```python
from build123d import *

# Parameters (mm, degrees)
ESBO_O1_W                     = 38
ESBO_O1_H                     = 56
ESBO_O1_R                     = 4
RESSALTO_EXTRUS_O1_DEPTH      = 6.4
ESBO_O6_R                     = 16.54
CORTE_EXTRUS_O5_DEPTH         = 4.6
ESBO_O7_R                     = 4
ESBO_O7_R_2                   = 1.25
CORTE_EXTRUS_O6_DEPTH         = 60.314079273
RESSALTO_EXTRUS_O2_DEPTH      = 4.6
RESSALTO_EXTRUS_O3_DEPTH      = 5.59
ESBO_O17_R                    = 3.5
RESSALTO_EXTRUS_O4_DEPTH      = 7
ESBO_O18_R                    = 2
RESSALTO_EXTRUS_O5_DEPTH      = 4
CHANFRO1_SIZE                 = 4
CHANFRO1_SIZE_2               = 5.29
FURO_ROSCADO_DE_M3X0_51_D     = 2.5
FURO_ROSCADO_DE_M3X0_51_DEPTH = 10
FURO_ROSCADO_DE_M3X0_51_TIP   = 0.751075774
CHANFRO2_SIZE                 = 1
SKETCH1_R                     = 1.25
CUT_EXTRUDE1_DEPTH            = 6
SKETCH2_R                     = 1.25
CUT_EXTRUDE2_DEPTH            = 10


# Read off the part's stored shape, not the designer's step: Escareado para parafuso de máquina com cabeça chata de M2.51
with BuildPart() as part:
    # Esboço1 → Ressalto-extrusão1 (new body)
    with BuildSketch(Plane.XY):
        with Locations((0, 28)):
            Rectangle(ESBO_O1_W, ESBO_O1_H)
        with Locations((0, 20)):
            Circle(ESBO_O1_R, mode=Mode.SUBTRACT)
    extrude(amount=RESSALTO_EXTRUS_O1_DEPTH)

    # Esboço6 → Corte-extrusão5 (cut)
    with BuildSketch(Plane(origin=(0, 0, 0), x_dir=(-1, 0, 0), z_dir=(0, 0, -1))):
        with Locations((0, 38.5)):
            Circle(ESBO_O6_R)
    extrude(amount=-CORTE_EXTRUS_O5_DEPTH, mode=Mode.SUBTRACT)

    # Esboço7 → Corte-extrusão6 (cut, through all)
    with BuildSketch(Plane(origin=(0, 0, 4.6), x_dir=(-1, 0, 0), z_dir=(0, 0, -1))):
        with Locations((0, 38.5)):
            Circle(ESBO_O7_R)
        with Locations((11.258330249, 32)):
            Circle(ESBO_O7_R_2)
        with Locations((-11.258330249, 32)):
            Circle(ESBO_O7_R_2)
        with Locations((0, 51.5)):
            Circle(ESBO_O7_R_2)
    extrude(amount=-CORTE_EXTRUS_O6_DEPTH, mode=Mode.SUBTRACT)

    # Escareado para parafuso de m_quina c 2 → Escareado para parafuso de máquina com cabeça chata de M2.51 (revolve, cut)
    with BuildSketch(Plane(origin=(-11.258330249, 32, 0), x_dir=(1, 0, 0), z_dir=(0, -1, 0))):
        Polygon((1.25, 4.6), (1.45, 4.6), (1.45, 5.1), (2.75, 6.4), (1.25, 6.4), align=None)
    revolve(axis=Axis((-11.258330249, 32, 0), (0, 0, 1)), mode=Mode.SUBTRACT)

    # Escareado para parafuso de m_quina c 3 o → Escareado para parafuso de m_quina c 3 (revolve, cut)
    with BuildSketch(Plane(origin=(11.258330249, 32, 0), x_dir=(1, 0, 0), z_dir=(0, -1, 0))):
        Polygon((1.25, 4.6), (1.45, 4.6), (1.45, 5.1), (2.75, 6.4), (1.25, 6.4), align=None)
    revolve(axis=Axis((11.258330249, 32, 0), (0, 0, 1)), mode=Mode.SUBTRACT)

    # Escareado para parafuso de m_quina c 4 o → Escareado para parafuso de m_quina c 4 (revolve, cut)
    with BuildSketch(Plane.XZ.offset(-51.5)):
        Polygon((1.25, 4.6), (1.45, 4.6), (1.45, 5.1), (2.75, 6.4), (1.25, 6.4), align=None)
    revolve(axis=Axis((0, 51.5, 0), (0, 0, 1)), mode=Mode.SUBTRACT)

    # Esboço15 → Ressalto-extrusão2 (add)
    with BuildSketch(Plane(origin=(0, 0, 0), x_dir=(-1, 0, 0), z_dir=(0, 0, -1))):
        with BuildLine():
            ThreePointArc((-3.280592218, 22.288605405), (0, 16), (3.280592218, 22.288605405))
            ThreePointArc((3.280592218, 22.288605405), (0, 21.96), (-3.280592218, 22.288605405))
        make_face()
    extrude(amount=-RESSALTO_EXTRUS_O2_DEPTH)

    # Esboço16 → Ressalto-extrusão3 (add)
    with BuildSketch(Plane.XY.offset(4.6)):
        with BuildLine():
            ThreePointArc((-3.280592218, 22.288605405), (0, 16), (3.280592218, 22.288605405))
            ThreePointArc((3.280592218, 22.288605405), (0, 24), (-3.280592218, 22.288605405))
        make_face()
    extrude(amount=RESSALTO_EXTRUS_O3_DEPTH)

    # Esboço17 → Ressalto-extrusão4 (add)
    with BuildSketch(Plane.XY.offset(10.19)):
        with Locations((0, 20)):
            Circle(ESBO_O17_R)
    extrude(amount=RESSALTO_EXTRUS_O4_DEPTH)

    # Esboço18 → Ressalto-extrusão5 (add)
    with BuildSketch(Plane.XY.offset(17.19)):
        with Locations((0, 20)):
            Circle(ESBO_O18_R)
    extrude(amount=RESSALTO_EXTRUS_O5_DEPTH)

    # Chanfro1
    # the kernel refuses this chamfer: 5.29, 4 mm, written as the material it adds along each edge
    with BuildSketch(Plane(origin=(0, 20, 6.4), x_dir=(0.8201480544065356, 0.5721513513513485, 0), z_dir=(-0.5721513513513485, 0.8201480544065356, 0))) as chanfro1_piece_1_section:
        Polygon((4 + CHANFRO1_SIZE, 0), (4, -CHANFRO1_SIZE_2), (4, 0), align=None)
    chanfro1_piece_1 = revolve(axis=Axis((0, 20, 6.4), (0, 0, -1)), mode=Mode.PRIVATE)
    chanfro1_piece_1 = split(chanfro1_piece_1, bisect_by=Plane(origin=(-5.391672128, 16.238663888, 10.19), z_dir=(0, 0, -1)), keep=Keep.TOP, mode=Mode.PRIVATE)
    add(chanfro1_piece_1)

    # Furo roscado de M3x0.51
    with Locations(Plane.XY.offset(21.19)):
        with Locations((0, 20)):
            Hole(FURO_ROSCADO_DE_M3X0_51_D / 2, depth=FURO_ROSCADO_DE_M3X0_51_DEPTH)
            with Locations((0, 0, -(FURO_ROSCADO_DE_M3X0_51_DEPTH + FURO_ROSCADO_DE_M3X0_51_TIP / 2))):  # 118° drill point
                Cone(0, FURO_ROSCADO_DE_M3X0_51_D / 2, FURO_ROSCADO_DE_M3X0_51_TIP, mode=Mode.SUBTRACT)

    # Chanfro2
    chanfro2_edges = [part.edges().sort_by_distance(p)[0] for p in [
        (4, 38.5, 6.4),
    ]]
    chamfer(chanfro2_edges, length=CHANFRO2_SIZE)

    # Sketch1 → Cut-Extrude1 (cut)
    with BuildSketch(Plane(origin=(0, 56, 0), x_dir=(1, 0, 0), z_dir=(0, 1, 0))):
        with Locations(Location((-14, -3, 0), (0, 0, 180))):
            Circle(SKETCH1_R)
        with Locations((14, -3)):
            Circle(SKETCH1_R)
    extrude(amount=-CUT_EXTRUDE1_DEPTH, mode=Mode.SUBTRACT)

    # Sketch2 → Cut-Extrude2 (cut)
    with BuildSketch(Plane(origin=(0, 0, 0), x_dir=(-1, 0, 0), z_dir=(0, -1, 0))):
        with Locations(Location((-12, -3, 0), (0, 0, 90))):
            Circle(SKETCH2_R)
        with Locations(Location((0, -3, 0), (0, 0, 90))):
            Circle(SKETCH2_R)
        with Locations(Location((12, -3, 0), (0, 0, 270))):
            Circle(SKETCH2_R)
    extrude(amount=-CUT_EXTRUDE2_DEPTH, mode=Mode.SUBTRACT)


solid = part.part
```
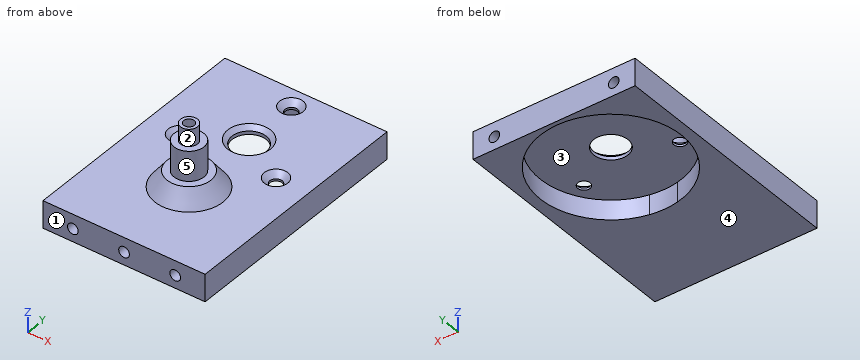
Source: CAD feature listing. Evaluate the final solid. Frame: model axes, mm. Face numbers are marked on the shaded views. A direction names the side the tool comes from. Coordinates: 2 decimals unless noted, no trailing zeros. Loops run counter-clockwise (first coordinate to the right, second up) from the corner with the lowest first, then second, coordinate; pieces in that order, holes last. Notation, with made-up numbers: M 89,-38.75 L 122,-38.75 A26 ccw 122,-12.75 Z; hole C 18,4.25 d11. An arc over 180 degrees is marked long. Use a Markdown table: item, result. Add a question column.
Q1. Section query C-C, the plane y = 32. Return loops of the section in (x, z).
Q2. Material intervals for L1, parallel to Y at x = 0, z = 4.75; L2, parallel to Z at x = -12, y = 3; L3, parallel to Y at x = 0, z = 14, sorted ascending.
Q3. Section query D-D, the plane y = 4.5. Return loops of the section in (x, z), and give its area (3 significant figures).
Q4. Draft query along Y for the marked faces 3, 4 and 5. Return one class per face: pulls with the +Y half, pulls with the -Y half, needs draft (parallel to the pull), parting line crosses it, or undercut.
Q5. Access query for the marked faces 1 and 2. Directions: +Z, -Z, +X, -X, +Y, -Y. A direction counts if a zero-diameter tool reaches every point of the face in a straight line with its end or side. Return the directions, or none.
Q6. Section query A-A, the plane z = 3. Return loops of the section in (x, y).
Q7. Section query B-B, the plane y = 51.5. Return loops of the section in (x, z), and give its area (3 significant figures).
Q8. First-contact query: pin 1 (8 mm diameter, centred on x = -5.5, z = 13, fed in from -Y); pin 2 (2 mm diameter, centred on x = 2.5, z = 12, fed in from +Y); pin 3 (2 mm diameter, centred on x = 12.5, z = 2.5, fed in from -Y); pin 4 (2 mm diameter, centred on x = 0, z = 3, fed in from -Y). Flat tips, straight axial feed; report the tip coordinate or a pass-through.
Result:
| question | item | result |
|---|---|---|
| 1 | outline | M -19,0 L -15.21,0 L -15.21,4.6 L -12.71,4.6 L -12.71,5.1 L -14.01,6.4 L -19,6.4 Z; M -9.81,4.6 L 9.81,4.6 L 9.81,5.1 L 8.51,6.4 L -8.51,6.4 L -9.81,5.1 Z; M 12.71,4.6 L 15.21,4.6 L 15.21,0 L 19,0 L 19,6.4 L 14.01,6.4 L 12.71,5.1 Z |
| 2 | L1 | y = 0 to 34.5, 42.5 to 50.05, 52.95 to 56 |
| 2 | L2 | z = 0 to 1.75, 4.25 to 6.4 |
| 2 | L3 | y = 16.5 to 18.75, 21.25 to 23.5 |
| 3 | outline | M -19,0 L 19,0 L 19,6.4 L -19,6.4 Z; hole C -12,3 d2.5; hole C 0,3 d2.5; hole C 12,3 d2.5 |
| 3 | area | 228 mm2 |
| 4 | face 3 | undercut |
| 4 | face 4 | needs draft |
| 4 | face 5 | parting line crosses it |
| 5 | face 1 | +Z, -Z, +X, -X, -Y |
| 5 | face 2 | +Z |
| 6 | outline | M -19,0 L -13.25,0 L -13.25,10 L -10.75,10 L -10.75,0 L -1.25,0 L -1.25,10 L 1.25,10 L 1.25,0 L 10.75,0 L 10.75,10 L 13.25,10 L 13.25,0 L 19,0 L 19,56 L 15.25,56 L 15.25,50 L 12.75,50 L 12.75,56 L -12.75,56 L -12.75,50 L -15.25,50 L -15.25,56 L -19,56 Z; hole C 0,38.5 d33.08 |
| 7 | outline | M -19,0 L -10.23,0 L -10.23,4.6 L -1.45,4.6 L -1.45,5.1 L -2.75,6.4 L -19,6.4 Z; M 1.45,4.6 L 10.23,4.6 L 10.23,0 L 19,0 L 19,6.4 L 2.75,6.4 L 1.45,5.1 Z; hole C -14,3 d2.5; hole C 14,3 d2.5 |
| 7 | area | 132 mm2 |
| 8 | pin 1 | stops at y = 15.54 |
| 8 | pin 2 | stops at y = 23.16 |
| 8 | pin 3 | stops at y = 0 |
| 8 | pin 4 | stops at y = 10 |
